```python
from build123d import *

# Parameters (mm, degrees)
BOSS_EXTRUDE1_DEPTH = 15.1
SKETCH2_W           = 20.2
SKETCH2_H           = 52.5
CUT_EXTRUDE1_DEPTH  = 39
SKETCH3_W           = 20.2
SKETCH3_H           = 12
CUT_EXTRUDE2_DEPTH  = 2.5
FILLET1_R           = 3
FILLET2_R           = 1.5
CUT_EXTRUDE3_REACH  = 50.613
SKETCH4_R           = 2
CUT_EXTRUDE4_DEPTH  = 2.5
CUT_EXTRUDE5_START  = -2.5
CUT_EXTRUDE5_DEPTH  = 2.5


with BuildPart() as part:
    # Sketch1 → Boss-Extrude1 (new, symmetric)
    with BuildSketch(Plane(origin=(0, 0, 0), x_dir=(0, 0, -1), z_dir=(1, 0, 0))):
        Polygon((-19.5, -27.5), (19.5, -27.5), (19.5, 27.5), (7.5, 27.5), (7.5, 37.5), (4, 37.5), (4, 27.5), (-4, 27.5), (-4, 37.5), (-7.5, 37.5), (-7.5, 27.5), (-19.5, 27.5), align=None)
    extrude(amount=BOSS_EXTRUDE1_DEPTH, both=True)

    # Sketch2 → Cut-Extrude1 (cut)
    with BuildSketch(Plane.XY.offset(19.5)):
        with Locations((0, -1.25)):
            Rectangle(SKETCH2_W, SKETCH2_H)
    extrude(amount=-CUT_EXTRUDE1_DEPTH, mode=Mode.SUBTRACT)

    # Sketch3 → Cut-Extrude2 (cut)
    with BuildSketch(Plane(origin=(0, 27.5, 0), x_dir=(1, 0, 0), z_dir=(0, 1, 0))):
        with Locations((0, -13.5)):
            Rectangle(SKETCH3_W, SKETCH3_H)
        with Locations((0, 13.5)):
            Rectangle(SKETCH3_W, SKETCH3_H)
    extrude(amount=-CUT_EXTRUDE2_DEPTH, mode=Mode.SUBTRACT)

    # Fillet1
    fillet1_edges = [part.edges().sort_by_distance(p)[0] for p in [
        (12.6, 27.5, 7.5),
        (12.6, 27.5, -7.5),
        (-12.6, 27.5, 7.5),
        (-12.6, 27.5, -7.5),
    ]]
    fillet(fillet1_edges, radius=FILLET1_R)

    # Fillet2
    fillet2_edges = [part.edges().sort_by_distance(p)[0] for p in [
        (15.1, 37.5, -5.75),
        (-15.1, 37.5, 5.75),
        (-15.1, 37.5, -5.75),
        (0, 37.5, 7.5),
        (0, 37.5, 4),
        (0, 37.5, -4),
        (0, 37.5, -7.5),
        (15.1, 37.5, 5.75),
    ]]
    fillet(fillet2_edges, radius=FILLET2_R)

    # Cut-Extrude3: up to this face of the body (flat: up to its plane)
    cut_extrude3_end = Plane(part.part.faces().sort_by_distance((0, 31.045634921, -7.5))[0])
    # Sketch4 → Cut-Extrude3 (cut, up to the picked face)
    with BuildSketch(Plane.XY.offset(7.5), mode=Mode.PRIVATE) as cut_extrude3_sk1:
        with Locations((-4.95, 30)):
            Circle(SKETCH4_R)
    cut_extrude3_tool1 = split(extrude(cut_extrude3_sk1.sketch, amount=-CUT_EXTRUDE3_REACH, mode=Mode.PRIVATE), bisect_by=cut_extrude3_end, keep=Keep.BOTH, mode=Mode.PRIVATE)
    # Sketch4 → Cut-Extrude3 (cut, up to the picked face)
    with BuildSketch(Plane.XY.offset(7.5), mode=Mode.PRIVATE) as cut_extrude3_sk2:
        with Locations(Location((4.95, 30, 0), (0, 0, 270))):
            Circle(SKETCH4_R)
    cut_extrude3_tool2 = split(extrude(cut_extrude3_sk2.sketch, amount=-CUT_EXTRUDE3_REACH, mode=Mode.PRIVATE), bisect_by=cut_extrude3_end, keep=Keep.BOTH, mode=Mode.PRIVATE)
    add(cut_extrude3_tool1.solids().sort_by(Axis((-4.95, 30, 7.5), (0, 0, -1)))[0], mode=Mode.SUBTRACT)
    add(cut_extrude3_tool2.solids().sort_by(Axis((4.95, 30, 7.5), (0, 0, -1)))[0], mode=Mode.SUBTRACT)

    # Sketch5 → Cut-Extrude4 (cut)
    with BuildSketch(Plane(origin=(15.1, 0, 0), x_dir=(0, 0, -1), z_dir=(1, 0, 0))):
        with BuildLine():
            Line((13.163699082, 10.394877926), (7.685662738, 2.028808489))
            ThreePointArc((7.685662738, 2.028808489), (6.717514421, 0), (7.685662738, -2.028808489))
            Line((7.685662738, -2.028808489), (13.163699082, -10.394877926))
            ThreePointArc((13.163699082, -10.394877926), (12.904698757, -12.904698757), (10.394877926, -13.163699082))
            Line((10.394877926, -13.163699082), (2.028808489, -7.685662738))
            ThreePointArc((2.028808489, -7.685662738), (0, -6.717514421), (-2.028808489, -7.685662738))
            Line((-2.028808489, -7.685662738), (-10.394877926, -13.163699082))
            ThreePointArc((-10.394877926, -13.163699082), (-12.904698757, -12.904698757), (-13.163699082, -10.394877926))
            Line((-13.163699082, -10.394877926), (-7.685662738, -2.028808489))
            ThreePointArc((-7.685662738, -2.028808489), (-6.717514421, 0), (-7.685662738, 2.028808489))
            Line((-7.685662738, 2.028808489), (-13.163699082, 10.394877926))
            ThreePointArc((-13.163699082, 10.394877926), (-12.904698757, 12.904698757), (-10.394877926, 13.163699082))
            Line((-10.394877926, 13.163699082), (-2.028808489, 7.685662738))
            ThreePointArc((-2.028808489, 7.685662738), (0, 6.717514421), (2.028808489, 7.685662738))
            Line((2.028808489, 7.685662738), (10.394877926, 13.163699082))
            ThreePointArc((10.394877926, 13.163699082), (12.904698757, 12.904698757), (13.163699082, 10.394877926))
        make_face()
    extrude(amount=-CUT_EXTRUDE4_DEPTH, mode=Mode.SUBTRACT)

    # Sketch6 → Cut-Extrude5 (cut)
    with BuildSketch(Plane.ZY.offset(15.1).offset(CUT_EXTRUDE5_START)):
        with BuildLine():
            Line((13.163699082, 10.394877926), (7.685662738, 2.028808489))
            ThreePointArc((7.685662738, 2.028808489), (6.717514421, 0), (7.685662738, -2.028808489))
            Line((7.685662738, -2.028808489), (13.163699082, -10.394877926))
            ThreePointArc((13.163699082, -10.394877926), (12.904698757, -12.904698757), (10.394877926, -13.163699082))
            Line((10.394877926, -13.163699082), (2.028808489, -7.685662738))
            ThreePointArc((2.028808489, -7.685662738), (0, -6.717514421), (-2.028808489, -7.685662738))
            Line((-2.028808489, -7.685662738), (-10.394877926, -13.163699082))
            ThreePointArc((-10.394877926, -13.163699082), (-12.904698757, -12.904698757), (-13.163699082, -10.394877926))
            Line((-13.163699082, -10.394877926), (-7.685662738, -2.028808489))
            ThreePointArc((-7.685662738, -2.028808489), (-6.717514421, 0), (-7.685662738, 2.028808489))
            Line((-7.685662738, 2.028808489), (-13.163699082, 10.394877926))
            ThreePointArc((-13.163699082, 10.394877926), (-12.904698757, 12.904698757), (-10.394877926, 13.163699082))
            Line((-10.394877926, 13.163699082), (-2.028808489, 7.685662738))
            ThreePointArc((-2.028808489, 7.685662738), (0, 6.717514421), (2.028808489, 7.685662738))
            Line((2.028808489, 7.685662738), (10.394877926, 13.163699082))
            ThreePointArc((10.394877926, 13.163699082), (12.904698757, 12.904698757), (13.163699082, 10.394877926))
        make_face()
    extrude(amount=CUT_EXTRUDE5_DEPTH, mode=Mode.SUBTRACT)


solid = part.part
```
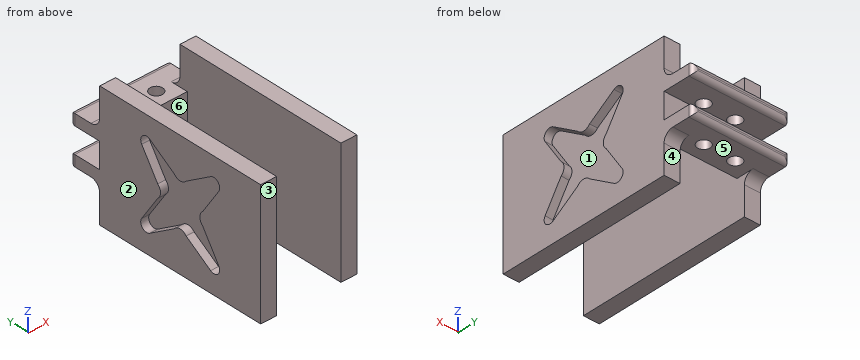
Geometry: final body of the model. Coordinates: model frame, mm. Face numbers are marked on the shaded views. A direction names the side the tool comes from. Coordinates: 2 decimals unless noted, no trailing zeros. Order: outer loops, then holes, each group sorted by start corner. A loop starts at its lowest first (then second) coordinate and runs counter-clockwise, first axis right, second up. Notation, with made-up numbers: (8.25, 38) -> (32.25, 38) arc R28 ccw to (32.25, 71) -> close; hole circle Ø7 at (-10.5, 45.25). An arc over 180 degrees is marked (long way). Write each question's results on one line, items separated by ' | '. Start each with the question number.
1) Cut plane D-D, the plane z = 0. Output: boundary loops of the cut face in (x, y).
2) Cut plane C-C, the plane x = -11. Output: boundary loops of the cut face in (y, z), and give its area (3 significant figures).
3) Set-up query: the marked faces 4, 5 and 6. Return all of +Z, -Z, +X, -X, +Y, -Y with unobstructed straight access to the full face (end or side cutting, diameter ignored); none if empty.
4) First-contact query: pin 1 (5.5 mm diameter, centred on x = 13, z = 13, fed in from +Y); pin 2 (3 mm diameter, centred on y = 10, z = 10, fed in from -X); pin 3 (9.5 mm diameter, centred on x = 2.5, y = 32.5, fed in from -Z). Flat tips, straight axial feed; report the tip coordinate or a pass-through.
5) Cut plane B-B, the plane x = -4.95. Output: boundary loops of the cut face in (y, z), and give its area (3 significant figures).
6) Cut plane A-A, the plane y = 23. Output: boundary loops of the cut face in (x, z), and give its area (3 significant figures).
7) Material intervals for line 1 along Z through (x, y) = (-8.5, 28); line 2 along X through (y, z) = (-10.5, -6); line 3 along X through (y, z) = (-8, 10), sorted ascending.
8) Mould query, pull axis Y, two halves, no side actions, for the marked faces 1, 2 and 3. Classes: released by +Y, released by -Y, zero draft, split by the parting line, or undercut.
Checks:
1) outline: (-15.1, -27.5) -> (-10.1, -27.5) -> (-10.1, 25) -> (10.1, 25) -> (10.1, -27.5) -> (15.1, -27.5) -> (15.1, -6.72) -> (12.6, -6.72) -> (12.6, 6.72) -> (15.1, 6.72) -> (15.1, 27.5) -> (-15.1, 27.5) -> (-15.1, 6.72) -> (-12.6, 6.72) -> (-12.6, -6.72) -> (-15.1, -6.72) -> close
2) outline: (-27.5, -19.5) -> (27.5, -19.5) -> (27.5, -10.5) arc R3 cw to (30.5, -7.5) -> (36, -7.5) arc R1.5 ccw to (37.5, -6) -> (37.5, -5.5) arc R1.5 ccw to (36, -4) -> (27.5, -4) -> (27.5, 4) -> (36, 4) arc R1.5 ccw to (37.5, 5.5) -> (37.5, 6) arc R1.5 ccw to (36, 7.5) -> (30.5, 7.5) arc R3 cw to (27.5, 10.5) -> (27.5, 19.5) -> (-27.5, 19.5) -> close | area: 2,220 mm^2
3) face 4: -Z, +X, -X, +Y | face 5: -Z, +Y | face 6: +Z, -Z, -Y
4) pin 1: y = 27.51 | pin 2: x = -12.6 | pin 3: z = -7.5
5) outline: (25, -7.5) -> (28, -7.5) -> (28, -4) -> (27.5, -4) -> (27.5, 4) -> (28, 4) -> (28, 7.5) -> (25, 7.5) -> close; (32, -7.5) -> (36, -7.5) arc R1.5 ccw to (37.5, -6) -> (37.5, -5.5) arc R1.5 ccw to (36, -4) -> (32, -4) -> close; (32, 4) -> (36, 4) arc R1.5 ccw to (37.5, 5.5) -> (37.5, 6) arc R1.5 ccw to (36, 7.5) -> (32, 7.5) -> close | area: 77.6 mm^2
6) outline: (-15.1, -19.5) -> (-10.1, -19.5) -> (-10.1, 19.5) -> (-15.1, 19.5) -> close; (10.1, -19.5) -> (15.1, -19.5) -> (15.1, 19.5) -> (10.1, 19.5) -> close | area: 390 mm^2
7) line 1: -7.5 to -4, 4 to 7.5 | line 2: -15.1 to -10.1, 10.1 to 15.1 | line 3: -12.6 to -10.1, 10.1 to 12.6
8) face 1: undercut | face 2: zero draft | face 3: released by -Y
